```python
from build123d import *

# Parameters (mm, degrees)
ESQUISSE1_W             = 5
ESQUISSE1_H             = 130
BOSS_EXTRU_1_DEPTH      = 15
CONG_1_R                = 8
ESQUISSE2_R             = 2.5
ENL_V_MAT_EXTRU_1_DEPTH = 15


with BuildPart() as part:
    # Esquisse1 → Boss.-Extru.1 (new body)
    with BuildSketch(Plane.XY):
        with Locations((2.5, 65)):
            Rectangle(ESQUISSE1_W, ESQUISSE1_H)
    extrude(amount=BOSS_EXTRU_1_DEPTH)

    # Congé1
    # the kernel refuses this fillet: 8 mm, written as the material it takes off along each edge
    with BuildSketch(Plane(origin=(-20, 0, 15), x_dir=(0, 0, -1), z_dir=(1, 0, 0)), Plane(origin=(25, 130, 15), x_dir=(0, 0, -1), z_dir=(-1, 0, 0))) as cong_1_piece_1:
        with BuildLine():
            CenterArc((CONG_1_R, CONG_1_R), CONG_1_R, 180, 90)
            Line((0, CONG_1_R), (0, 0))
            Line((0, 0), (CONG_1_R, 0))
        make_face()
    extrude(amount=45, mode=Mode.SUBTRACT)
    with BuildSketch(Plane(origin=(-20, 0, 0), x_dir=(0, 0, 1), z_dir=(1, 0, 0)), Plane(origin=(25, 130, 0), x_dir=(0, 0, 1), z_dir=(-1, 0, 0))) as cong_1_piece_2:
        with BuildLine():
            CenterArc((CONG_1_R, -CONG_1_R), CONG_1_R, 90, 90)
            Line((0, -CONG_1_R), (0, 0))
            Line((0, 0), (CONG_1_R, 0))
        make_face()
    extrude(amount=45, mode=Mode.SUBTRACT)

    # Esquisse2 → Enlèv. mat.-Extru.1 (cut)
    with BuildSketch(Plane(origin=(5, 0, 0), x_dir=(0, 0, -1), z_dir=(1, 0, 0))):
        with Locations((-7, 122)):
            Circle(ESQUISSE2_R)
        with Locations((-8, 8)):
            Circle(ESQUISSE2_R)
    extrude(amount=-ENL_V_MAT_EXTRU_1_DEPTH, mode=Mode.SUBTRACT)


solid = part.part
```
Here's how the part is built. I have some questions about the finished solid (model axes, mm). Give positions to 0.01 mm unless a question says otherwise; leave off trailing zeros. Loops run counter-clockwise (first coordinate to the right, second up) from the corner with the lowest first, then second, coordinate; pieces in that order, holes last. Notation, with made-up numbers: M 38,39 L 90,39 A23 ccw 90,75 Z; hole C -36.5,29.5 d7. An arc over 180 degrees is marked long. Put each result on its own line as item: value. Start each with the question number.
(1) I want a section at B-B on z = 1.75. Please give me the cut outline in (x, y), then the cut area to 3 significant figures.
(2) I need wall thicknesses on line 1 along Y through (x, z) = (2.7, 7); line 2 along Y through (x, z) = (3.5, 8); line 3 along Y through (x, z) = (0.75, 10). Which ranges of each line are inside material? Lowest first, please. Write a range as [from, to].
(3) If we mould it in two halves opening along Y, with no side actions, what happens to faces 1 (the flat face through (2, 66, 0)), 2 (the cylindrical face through (2.54, 5.56, 8.54)), 3 (the cylindrical face through (2.54, 127.54, 2.23))? For each: +Y half, -Y half, draft (parallel to the pull), parting line (faces both ways), or undercut.
(4) I want a section at A-A on x = 2.35. Please give me the cut outline in (y, z).
(5) Will these pins go through, and if not, where does the flat tip stop? pin 1 Ø6.5 at (y, z) = (122, 7) entering from -X; pin 2 Ø1.5 at (x, z) = (3, 1.5) entering from +Y.
Answer block:
1. outline: M 0,3.01 L 5,3.01 L 5,126.99 L 0,126.99 Z
1. area: 620 mm^2
2. line 1: [0.06, 5.71], [10.29, 119.5], [124.5, 129.94]
2. line 2: [0.06, 5.5], [10.5, 119.71], [124.29, 129.94]
2. line 3: [0.58, 6.5], [9.5, 129.42]
3. face 1: draft
3. face 2: undercut
3. face 3: +Y half
4. outline: M 0.02,7.5 A8 ccw 8,0 L 122,0 A8 ccw 129.98,7.5 A8 ccw 122,15 L 8,15 A8 ccw Z; hole C 8,8 d5; hole C 122,7 d5
5. pin 1: x = 0
5. pin 2: y = 127.56
